from build123d import *

# Parameters (mm, degrees)
F2_R     = 1.524
F4_D     = 7.9375
F4_DEPTH = 23.8125
F4_TIP   = 2.3846655818
F5_SIZE  = 1.524


with BuildPart() as f1:
    # F0 (on Right) → F1 (revolve)
    with BuildSketch(Plane.YZ):
        Polygon((-228.6, 0), (0, 0), (0, 10), (-203.1287532383, 10), (-228.6, 3.175), align=None)
    revolve(axis=Axis((0, -114.3, 0), (0, -1, 0)))

    # F2
    f2_edges = [f1.edges().sort_by_distance(p)[0] for p in [
        (0, -203.128753, -10),
        (0, -228.6, -3.175),
    ]]
    fillet(f2_edges, radius=F2_R)

    # F4
    with Locations(Plane(origin=(0, 0, 0), x_dir=(-1, 0, 0), z_dir=(0, 1, 0))):
        with Locations((0, 0)):
            Hole(F4_D / 2, depth=F4_DEPTH)
            with Locations((0, 0, -(F4_DEPTH + F4_TIP / 2))):  # 118° drill point
                Cone(0, F4_D / 2, F4_TIP, mode=Mode.SUBTRACT)

    # F5
    f5_edges = [f1.edges().sort_by_distance(p)[0] for p in [
        (0, 0, -10),
    ]]
    chamfer(f5_edges, length=F5_SIZE)


solid = f1.part
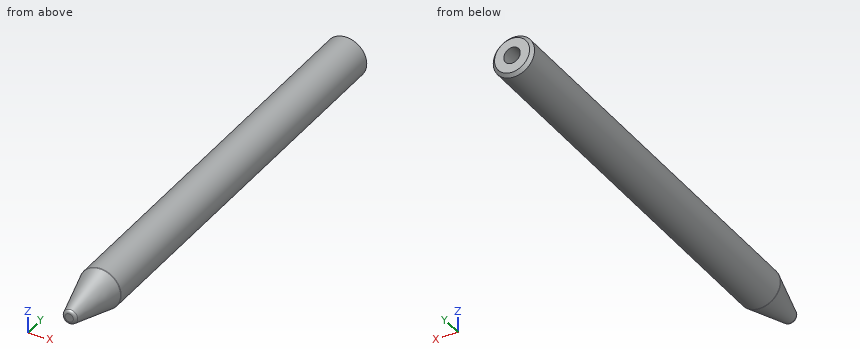
Design review of the part built by this model. Coordinates are the model's own, in mm. Round coordinates to 2 decimals unless told otherwise and drop trailing zeros. Order: outer loops, then holes, each group sorted by start corner. A loop starts at its lowest first (then second) coordinate and runs counter-clockwise, first axis right, second up.
1) Consider section A-A (y = -21). State the section outline as (x, z) points.
The answers:
outline: circle Ø20 at (0, 0); hole circle Ø7.94 at (0, 0)
2) Clearance check with flat-ended pins moving along their axes: pin 1 Ø6 at (y, z) = (-188, -4) entering from +X; pin 2 Ø3 at (y, z) = (-23, 7) entering from +X; pin 3 Ø1 at (x, y) = (2, -106) entering from +Z. State where each tip first meets the part, or that it passes through.
The answers:
pin 1: stops at x = 9.95
pin 2: stops at x = 8.35
pin 3: stops at z = 9.89
3) Consider section B-B (y = -68). State the section outline as (x, z) points.
The answers:
outline: circle Ø20 at (0, 0)
4) For L1, parallel to X at y = -12.75, z = 0; L2, parallel to Y at x = 3, z = -0.5, list the stretches that pass through material, from the lowest coordinate up.
The answers:
L1: x = -10 to -3.97, 3.97 to 10
L2: y = -228.19 to -24.37
